from build123d import *

# Parameters (mm, degrees)
SKETCH1_W           = 155
SKETCH1_H           = 40
BOSS_EXTRUDE1_DEPTH = 0.5
SKETCH2_W           = 160
SKETCH2_H           = 45
SKETCH2_W_2         = 155
SKETCH2_H_2         = 40
BOSS_EXTRUDE2_DEPTH = 4
FILLET1_R           = 1
SKETCH3_W           = 164
SKETCH3_H           = 49
BOSS_EXTRUDE3_DEPTH = 0.5
SKETCH5_R           = 3.5
SKETCH5_R_2         = 4.75
SKETCH5_W           = 13
SKETCH5_H           = 6.25
SKETCH5_W_2         = 10
SKETCH5_H_2         = 4
CUT_EXTRUDE1_DEPTH  = 86.653371212
CUT_EXTRUDE2_DEPTH  = 86.653371212


with BuildPart() as part:
    # Sketch1 → Boss-Extrude1 (new body)
    with BuildSketch(Plane(origin=(0, 0, 0), x_dir=(1, 0, 0), z_dir=(0, 1, 0))):
        Rectangle(SKETCH1_W, SKETCH1_H)
    extrude(amount=BOSS_EXTRUDE1_DEPTH)

    # Sketch2 → Boss-Extrude2 (add)
    with BuildSketch(Plane.XZ):
        Rectangle(SKETCH2_W, SKETCH2_H)
        Rectangle(SKETCH2_W_2, SKETCH2_H_2, mode=Mode.SUBTRACT)
    extrude(amount=-BOSS_EXTRUDE2_DEPTH)

    # Fillet1
    fillet1_edges = [part.edges().sort_by_distance(p)[0] for p in [
        (-80, 4, 0),
        (0, 4, 22.5),
        (80, 4, 0),
        (0, 4, -22.5),
        (77.5, 4, 0),
        (0, 4, 20),
        (-77.5, 4, 0),
        (0, 4, -20),
    ]]
    fillet(fillet1_edges, radius=FILLET1_R)

    # Sketch3 → Boss-Extrude3 (add)
    with BuildSketch(Plane.XZ):
        Rectangle(SKETCH3_W, SKETCH3_H)
    extrude(amount=-BOSS_EXTRUDE3_DEPTH)

    # Sketch5 → Cut-Extrude1 (cut, through all)
    with BuildSketch(Plane(origin=(0, 0.5, 0), x_dir=(1, 0, 0), z_dir=(0, 1, 0))):
        with Locations(Location((74, 13.5, 0), (0, 0, 270))):
            Circle(SKETCH5_R)
        with Locations(Location((63.5, 13.5, 0), (0, 0, 270))):
            Circle(SKETCH5_R)
        with Locations(Location((53, 13.5, 0), (0, 0, 270))):
            Circle(SKETCH5_R)
        with Locations(Location((40.75, 12.25, 0), (0, 0, 270))):
            Circle(SKETCH5_R_2)
        with Locations(Location((40.75, -10.75, 0), (0, 0, 270))):
            Circle(SKETCH5_R_2)
        with Locations((21.5, -13.875)):
            Rectangle(SKETCH5_W, SKETCH5_H)
        with Locations((21.5, -5.125)):
            Rectangle(SKETCH5_W, SKETCH5_H)
        Polygon((13, 11), (13, 9), (15, 9), (15, 1), (28, 1), (28, 9), (30, 9), (30, 11), align=None)
        with Locations((-0.5, -13.875)):
            Rectangle(SKETCH5_W, SKETCH5_H)
        with Locations((-0.5, -5.225)):
            Rectangle(SKETCH5_W, SKETCH5_H)
        with Locations((-0.5, 3.425)):
            Rectangle(SKETCH5_W, SKETCH5_H)
        with Locations((-0.5, 12.075)):
            Rectangle(SKETCH5_W, SKETCH5_H)
        with Locations((-23.389803957, -5.875)):
            Rectangle(SKETCH5_W, SKETCH5_H)
        with Locations((-23.389803957, -15)):
            Rectangle(SKETCH5_W_2, SKETCH5_H_2)
        Polygon((-55.5, 3), (-55.5, -1), (-53.75, -3.25), (-38.25, -3.25), (-38.25, 3), align=None)
        Polygon((-39.125, -12.25), (-39.125, -16.25), (-41.375, -18.25), (-52.375, -18.25), (-54.625, -16.25), (-54.625, -12.25), align=None)
    extrude(amount=-CUT_EXTRUDE1_DEPTH, mode=Mode.SUBTRACT)

    # Sketch7 → Cut-Extrude2 (cut, through all)
    with BuildSketch(Plane(origin=(0, 0.5, 0), x_dir=(1, 0, 0), z_dir=(0, 1, 0))):
        Polygon((-67.250510445, 14.746570529), (-64.239153938, 14.746570529), (-70.176868986, 8.808855481), (-73.200368059, 8.808855481), align=None)
        Polygon((-61.640644694, 14.746570529), (-58.726428719, 14.746570529), (-62.859039574, 10.622393574), (-65.744832191, 10.622393574), align=None)
        Polygon((-55.885068144, 14.746570529), (-53.165133234, 14.746570529), (-60.336027284, 7.540750618), (-63.437744545, 7.540750618), align=None)
        Polygon((-50.323772659, 14.746570529), (-47.409556685, 14.746570529), (-53.318492244, 8.808855481), (-56.346485673, 8.808855481), align=None)
        Polygon((-44.738192041, 14.746570529), (-41.896831466, 14.746570529), (-46.335248567, 10.37079238), (-49.279511935, 10.37079238), align=None)
        Polygon((-50.736619922, 8.808855481), (-47.807380251, 8.808855481), (-50.607399688, 6.110903309), (-53.686609439, 6.110903309), align=None)
        Polygon((-39.225466823, 14.746570529), (-36.262680582, 14.746570529), (-43.414652286, 7.594598825), (-46.335248567, 7.594598825), align=None)
        Polygon((-33.567030806, 14.746570529), (-30.774240497, 14.746570529), (-36.262680582, 9.225561643), (-39.225466823, 9.225561643), (-33.737026738, 14.746570529), align=None)
        Polygon((-28.039824293, 14.746570529), (-25.014130416, 14.746570529), (-31.833017792, 7.887219381), (-34.916396501, 7.887219381), align=None)
        Polygon((-22.574054709, 14.746570529), (-19.580895175, 14.746570529), (-21.648041016, 12.684601459), (-24.461046589, 12.684601459), align=None)
        Polygon((-25.957626356, 11.170584677), (-23.054543803, 11.170584677), (-31.544128494, 2.702260527), (-34.562960016, 2.702260527), align=None)
        Polygon((-27.096328353, 4.41957859), (-24.11943599, 4.41957859), (-20.893046917, 7.594598825), (-24.11943599, 7.594598825), align=None)
        Polygon((-22.378761422, 9.104350792), (-19.450757804, 9.104350792), (-13.809696196, 14.65559844), (-17.059483611, 14.65559844), align=None)
        Polygon((-23.898512836, 1.421313419), (-21.077474942, 1.328401476), (-10.722527867, 11.518482635), (-13.809696196, 11.518482635), align=None)
        Polygon((-17.270956838, 1.784296826), (-14.164624085, 1.784296826), (-10.489423725, 5.462539901), (-10.489423725, 8.583974463), align=None)
        Polygon((45.285967662, 3.623418363), (45.285967662, 0.513302694), (49.202811749, 4.367784889), (46.145186604, 4.367784889), align=None)
        Polygon((45.285967662, -2.026996785), (45.285967662, -3.633362633), (46.817618819, -3.633362633), (54.819393397, 4.241011979), (51.562001671, 4.241011979), align=None)
        Polygon((51.188428218, -1.877567404), (53.990229114, -1.877567404), (60.195561112, 4.319829757), (57.092895113, 4.319829757), align=None)
        Polygon((50.067707859, -8.508496193), (53.057358815, -8.606961469), (66.000700856, 4.319829757), (62.750526584, 4.319829757), align=None)
        Polygon((68.242056341, 4.319829757), (71.305358655, 4.319829757), (60.033658541, -7.081188124), (57.092895113, -7.081188124), align=None)
        Polygon((74.235786126, 4.241011979), (75.951599175, 4.241011979), (75.951599175, 2.702260527), (71.305358655, -2.048937359), (68.051709926, -2.048937359), align=None)
        Polygon((75.808614755, -1.231673392), (75.808614755, -4.252219282), (73.574483179, -6.486350857), (70.518191185, -6.486350857), (75.772868649, -1.231673392), align=None)
        Polygon((75.808614755, -7.969814223), (75.808614755, -10.883121797), (70.518191185, -16.173545367), (67.354660874, -16.173545367), align=None)
        Polygon((69.088346976, -7.665972329), (72.305496445, -7.665972329), (65.603005834, -14.36846294), (62.475317514, -14.36846294), align=None)
        Polygon((66.621865717, -3.251328336), (69.981999606, -3.251328336), (57.399370575, -15.619480737), (54.200094159, -15.619480737), align=None)
    extrude(amount=-CUT_EXTRUDE2_DEPTH, mode=Mode.SUBTRACT)


solid = part.part
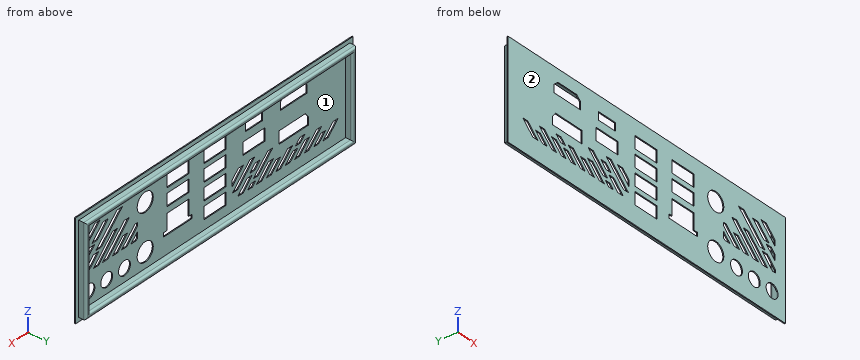
The model under review builds one solid part; all positions refer to its coordinate system, in mm. Face numbers are marked on the shaded views. Round coordinates to 2 decimals unless told otherwise and drop trailing zeros. Loops run counter-clockwise (first coordinate to the right, second up) from the corner with the lowest first, then second, coordinate; pieces in that order, holes last. Notation, with made-up numbers: M 31.25,-9.75 L 69.25,-9.75 A8 cw 69.25,3.25 Z; hole C 2.5,31 d8. An arc over 180 degrees is marked long. Answer as a JSON object with one key per item and string values.
Item 1: The part is to be moulded in two halves that separate along X. For the marked faces 1 and 2, say which applies: +X half, -X half, draft (parallel to the pull), parting line (faces both ways), or undercut.
Check sheet entries:
{"face 1": "undercut", "face 2": "draft"}
Item 2: Clearance check with flat-ended pins moving along their axes: P1, Ø12, axis at x = -40.5, z = -11, coming from the -Y side; P2, Ø11, axis at x = 53, z = -13.5, coming from the +Y side; P3, Ø1.2, axis at x = -37.5, y = 2, coming from the -Z side. State where each tip first meets the part, or that it passes through.
Check sheet entries:
{"P1": "y = 0", "P2": "y = 0.5", "P3": "z = -22.5"}
Item 3: We need section A-A, the plane y = 2.4. State the section outline as (x, z) points, and give its area (3 significant figures).
Check sheet entries:
{"outline": "M -80,-22.5 L 80,-22.5 L 80,22.5 L -80,22.5 Z; hole M -77.5,-20 L 77.5,-20 L 77.5,20 L -77.5,20 Z", "area": "1,000 mm2"}
Item 4: For line 1 along Z through (x, y) = (-1.5, 2.3); line 2 along Z through (x, y) = (18, 0.45); line 3 along X through (y, z) = (0.6, -2), list the stretches that pass through material, from the lowest coordinate up.
Check sheet entries:
{"line 1": "-22.5 to -20, 20 to 22.5", "line 2": "-24.5 to -11, -1 to 2, 8.25 to 10.75, 17 to 24.5", "line 3": "-80 to -77.5, 77.5 to 80"}
